from build123d import *

# Parameters (mm, degrees)
SKETCH1_R           = 10
BOSS_EXTRUDE1_DEPTH = 10
FILLET1_R           = 20


with BuildPart() as part:
    # Sketch1 → Boss-Extrude1 (new, symmetric)
    with BuildSketch(Plane(origin=(0, 0, 0), x_dir=(-1, 0, 0), z_dir=(0, 1, 0))):
        Polygon((-70, 0), (70, 0), (70, 10), (30, 10), (30, 60), (-30, 60), (-30, 10), (-70, 10), align=None)
        with Locations(Location((0, 30, 0), (0, 0, 90))):
            Circle(SKETCH1_R, mode=Mode.SUBTRACT)
    extrude(amount=BOSS_EXTRUDE1_DEPTH, both=True)

    # Fillet1
    fillet1_edges = [part.edges().sort_by_distance(p)[0] for p in [
        (30, 0, 60),
        (-30, 0, 60),
    ]]
    fillet(fillet1_edges, radius=FILLET1_R)


solid = part.part
Could you check a few things on this model? Use its own coordinates, in mm. A direction names the side the tool comes from. Give positions to 0.01 mm unless a question says otherwise; leave off trailing zeros. Loops run counter-clockwise (first coordinate to the right, second up) from the corner with the lowest first, then second, coordinate; pieces in that order, holes last. Notation, with made-up numbers: M -29,76 L -5,76 A22 cw -5,98 Z; hole C 89,16.5 d7. An arc over 180 degrees is marked long. Answer as a JSON object with one key per item and string values.
Q1. Suppose I cut it at A-A, the plane x = 0. List the corners of the cut face in (y, z) for me, plus the area to 3 significant figures.
Values found:
{"outline": "M -10,0 L 10,0 L 10,20 L -10,20 Z; M -10,40 L 10,40 L 10,60 L -10,60 Z", "area": "800 mm²"}
Q2. If we mould it in two halves opening along X, with no side actions, what happens to faces 4 (the flat face through (-30, 0, 25)), 5 (the cylindrical face through (3, -0.14, 39.54)), 6 (the cylindrical face through (24.297, -0.14, 53.986))? For each: pulls with the +X half, pulls with the -X half, needs draft (parallel to the pull), parting line crosses it, or undercut.
Values found:
{"face 4": "pulls with the -X half", "face 5": "undercut", "face 6": "pulls with the +X half"}
Q3. Suppose I cut it at D-D, the plane x = 37. List the corners of the cut face in (y, z) for me.
Values found:
{"outline": "M -10,0 L 10,0 L 10,10 L -10,10 Z"}
Q4. If I drill on probe 1 along X at (y, z) = (1, 30); probe 2 along X at (y, z) = (-4.5, 13.5); probe 3 along X at (y, z) = (-3.5, 28), over which ranges is the centre line in solid material (lowest first)? Write a range as [from, to].
Values found:
{"probe 1": "x = [-30, -10], [10, 30]", "probe 2": "x = [-30, 30]", "probe 3": "x = [-30, -9.8], [9.8, 30]"}
Q5. Suppose I cut it at B-B, the plane z = 30. List the corners of the cut face in (x, y) for me, plus the area to 3 significant figures.
Values found:
{"outline": "M -30,-10 L -10,-10 L -10,10 L -30,10 Z; M 10,-10 L 30,-10 L 30,10 L 10,10 Z", "area": "800 mm²"}
Q6. For P1, Ø1.5, axis at y = -7, z = 24, coming from the +X side; P2, Ø6, axis at y = 3, z = 25.5, coming from the -X side; P3, Ø12, axis at x = -52.5, y = 0.5, coming from the +Z side, each with a flat end and sliding along its axis, tell me the tip position at first contact or that it passes through.
Values found:
{"P1": "stops at x = 30", "P2": "stops at x = -30", "P3": "stops at z = 10"}
Q7. Suppose I cut it at C-C, the plane y = -8. List the corners of the cut face in (x, z) for me, plus the area to 3 significant figures.
Values found:
{"outline": "M -70,0 L 70,0 L 70,10 L 30,10 L 30,40 A20 ccw 10,60 L -10,60 A20 ccw -30,40 L -30,10 L -70,10 Z; hole C 0,30 d20", "area": "3,910 mm²"}
Q8. For faces 1 (the flat face through (-50, 0, 10)), 2 (the flat face through (30, 0, 25)), 3 (the flat face through (-70, 0, 5)), which set-ups out of +Z, -Z, +X, -X, +Y, -Y let a thin tool reach every point of the face, with its end or its side?
Values found:
{"face 1": "+Z, -X, +Y, -Y", "face 2": "+Z, +X, +Y, -Y", "face 3": "+Z, -Z, -X, +Y, -Y"}
